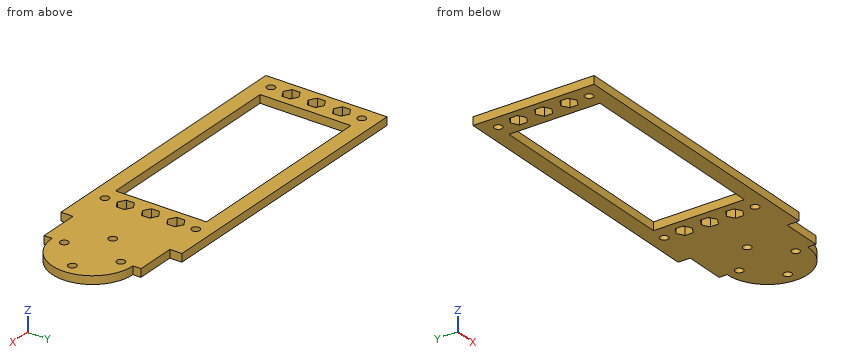
```python
from build123d import *

# Parameters (mm, degrees)
SKETCH1_R           = 1
SKETCH1_W           = 50
SKETCH1_H           = 22.5
BOSS_EXTRUDE1_DEPTH = 2


with BuildPart() as part:
    # Sketch1 → Boss-Extrude1 (new body)
    with BuildSketch(Plane.XY):
        with BuildLine():
            Line((0, 10), (0, 12))
            Line((0, 12), (-10, 12))
            Line((-10, 12), (-10, 15))
            Line((-10, 15), (-81, 15))
            Line((-81, 15), (-81, -15))
            Line((-81, -15), (-10, -15))
            Line((-10, -15), (-10, -12))
            Line((-10, -12), (0, -12))
            Line((0, -12), (0, -10))
            ThreePointArc((0, -10), (10, 0), (0, 10))
        make_face()
        with Locations((0, 7)):
            Circle(SKETCH1_R, mode=Mode.SUBTRACT)
        with Locations((7, 0)):
            Circle(SKETCH1_R, mode=Mode.SUBTRACT)
        with Locations((0, -7)):
            Circle(SKETCH1_R, mode=Mode.SUBTRACT)
        with Locations((-7, 0)):
            Circle(SKETCH1_R, mode=Mode.SUBTRACT)
        with Locations((-20, 11.25)):
            Circle(SKETCH1_R, mode=Mode.SUBTRACT)
        with Locations((-20, -11.25)):
            Circle(SKETCH1_R, mode=Mode.SUBTRACT)
        with Locations((-77.5, 11.25)):
            Circle(SKETCH1_R, mode=Mode.SUBTRACT)
        with Locations((-77.5, -11.25)):
            Circle(SKETCH1_R, mode=Mode.SUBTRACT)
        with Locations((-48.75, 0)):
            Rectangle(SKETCH1_W, SKETCH1_H, mode=Mode.SUBTRACT)
        Polygon((-20.096394859, 8.25), (-21.828445667, 7.25), (-21.828445667, 5.25), (-20.096394859, 4.25), (-18.364344051, 5.25), (-18.364344051, 7.25), align=None, mode=Mode.SUBTRACT)
        Polygon((-20.096394859, -8.25), (-18.364344051, -7.25), (-18.364344051, -5.25), (-20.096394859, -4.25), (-21.828445667, -5.25), (-21.828445667, -7.25), align=None, mode=Mode.SUBTRACT)
        Polygon((-20.096394859, -2), (-18.364344051, -1), (-18.364344051, 1), (-20.096394859, 2), (-21.828445667, 1), (-21.828445667, -1), align=None, mode=Mode.SUBTRACT)
        Polygon((-77.5, 4.25), (-75.767949192, 5.25), (-75.767949192, 7.25), (-77.5, 8.25), (-79.232050808, 7.25), (-79.232050808, 5.25), align=None, mode=Mode.SUBTRACT)
        Polygon((-77.5, -8.25), (-75.767949192, -7.25), (-75.767949192, -5.25), (-77.5, -4.25), (-79.232050808, -5.25), (-79.232050808, -7.25), align=None, mode=Mode.SUBTRACT)
        Polygon((-77.5, -2), (-75.767949192, -1), (-75.767949192, 1), (-77.5, 2), (-79.232050808, 1), (-79.232050808, -1), align=None, mode=Mode.SUBTRACT)
    extrude(amount=BOSS_EXTRUDE1_DEPTH)


solid = part.part
```
Work out the finished part from the listing and answer in its coordinate system (mm). Give positions to 0.01 mm unless a question says otherwise; leave off trailing zeros. Loops run counter-clockwise (first coordinate to the right, second up) from the corner with the lowest first, then second, coordinate; pieces in that order, holes last. Notation, with made-up numbers: (-17.5, 75.25) - (0.5, 75.25) arc R26 ccw to (0.5, 113.25) - close; hole circle Ø3 at (-13, -9). An arc over 180 degrees is marked (long way). Use CSV: the item, a comma, the result in double quotes. Start each with the question number.
(1) Find the intervals of material crossed by L1, parallel to Y at x = -77.5, z = 1.25; L2, parallel to Y at x = -57, z = 1.85; L3, parallel to X at y = -0.5, z = 1.1, in increasing order.
(2) Find section D-D, the plane z = 1.4. Count the separate pieces of the cut face and the enclosed holes in it, plus the area to 3 significant figures.
(3) Each of these flat-tipped pins is pushed along its axis until it touches: pin 1 (1 mm diameter, centred on y = -6.5, z = 1.5, fed in from +X); pin 2 (0.6 mm diameter, centred on y = 11, z = 1, fed in from +X). Where does it stop, or does it pass through?
(4) Find section B-B, the plane y = 0. Determine the outline of the cut face in (x, z).
(5) Find section A-A, the plane x = -7. Determine the outline of the cut face in (y, z).
(6) Find section C-C, the plane x = -27.5. Determine the outline of the cut face in (y, z).
Results found:
1,L1,"-15 to -12.25, -10.25 to -8.25, -4.25 to -2, 2 to 4.25, 8.25 to 10.25, 12.25 to 15"
1,L2,"-15 to -11.25, 11.25 to 15"
1,L3,"-81 to -79.23, -75.77 to -73.75, -23.75 to -21.83, -18.36 to -7.87, -6.13 to 6.13, 7.87 to 9.99"
2,separate pieces,"1"
2,enclosed holes,"15"
2,area,"1,310 mm^2"
3,pin 1,"x = 8"
3,pin 2,"x = 0"
4,outline,"(-81, 0) - (-79.23, 0) - (-79.23, 2) - (-81, 2) - close; (-75.77, 0) - (-73.75, 0) - (-73.75, 2) - (-75.77, 2) - close; (-23.75, 0) - (-21.83, 0) - (-21.83, 2) - (-23.75, 2) - close; (-18.36, 0) - (-8, 0) - (-8, 2) - (-18.36, 2) - close; (-6, 0) - (6, 0) - (6, 2) - (-6, 2) - close; (8, 0) - (10, 0) - (10, 2) - (8, 2) - close"
5,outline,"(-12, 0) - (-1, 0) - (-1, 2) - (-12, 2) - close; (1, 0) - (12, 0) - (12, 2) - (1, 2) - close"
6,outline,"(-15, 0) - (-11.25, 0) - (-11.25, 2) - (-15, 2) - close; (11.25, 0) - (15, 0) - (15, 2) - (11.25, 2) - close"
